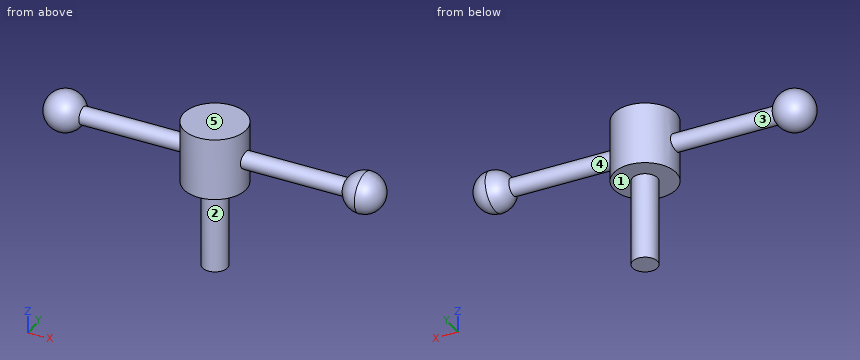
from build123d import *

# Parameters (mm, degrees)
F0_R     = 15.875
F1_DEPTH = 31.75
F2_R     = 6.35
F3_DEPTH = 44.45
F4_R     = 4.445
F5_DEPTH = 76.2


with BuildPart() as f1:
    # F0 (on Top) → F1 (new body)
    with BuildSketch(Plane.XY):
        Circle(F0_R)
    extrude(amount=F1_DEPTH)

    # F2 (on face) → F3 (join)
    with BuildSketch(Plane(origin=(0, 0, 0), x_dir=(1, 0, 0), z_dir=(0, 0, -1))):
        Circle(F2_R)
    extrude(amount=F3_DEPTH)

    # F4 (on Right) → F5 (join, symmetric)
    with BuildSketch(Plane.YZ):
        with Locations((0, 15.875)):
            Circle(F4_R)
    extrude(amount=F5_DEPTH, both=True)

    # F6 (on Front) → F7 (revolve)
    with BuildSketch(Plane.XZ):
        with BuildLine():
            Line((-76.2, 15.875), (-76.2, 20.32))
            Line((-76.2, 20.32), (-67.063941, 20.32))
            ThreePointArc((-67.063941, 20.32), (-78.480706, 25.775706), (-86.36, 15.875))
            Line((-86.36, 15.875), (-76.2, 15.875))
        make_face()
        with BuildLine():
            Line((76.2, 26.035), (76.2, 20.32))
            Line((76.2, 20.32), (76.2, 15.875))
            Line((76.2, 15.875), (86.36, 15.875))
            ThreePointArc((86.36, 15.875), (83.384205, 23.059205), (76.2, 26.035))
        make_face()
        with BuildLine():
            ThreePointArc((76.2, 26.035), (70.811846, 24.488559), (67.063941, 20.32))
            Line((67.063941, 20.32), (76.2, 20.32))
            Line((76.2, 20.32), (76.2, 26.035))
        make_face()
    revolve(axis=Axis((-81.28, 0, 15.875), (1, 0, 0)))


solid = f1.part
For this review, take the finished solid that the model builds, in its own axes (mm). Face numbers are marked on the shaded views. A direction names the side the tool comes from. Round coordinates to 2 decimals unless told otherwise and drop trailing zeros. Write each loop counter-clockwise with the first axis right and the second up, starting at its lowest first coordinate (ties: lowest second). Pieces come first, ordered by that corner, then holes. Notation, with made-up numbers: (10.25, -25) -> (32.25, -25) arc R37 cw to (32.25, 11) -> close; hole circle Ø3 at (-31.5, 38.25). An arc over 180 degrees is marked (long way). Put each result on its own line as item: value.
Q1. Consider section B-B on z = 3. State the section outline as (x, y) points (3 decimals), and give its area (3 significant figures).
Determined:
outline: circle Ø31.75 at (0, 0)
area: 792 mm^2
Q2. Consider section D-D on x = -39.5. State the section outline as (y, z) points (3 decimals).
Determined:
outline: circle Ø8.89 at (0, 15.875)
Q3. Clearance check with flat-ended pins moving along their axes: pin 1 Ø10 at (x, y) = (63.5, -3.5) entering from +Z; pin 2 Ø10 at (x, y) = (-54, 9) entering from -Z; pin 3 Ø2 at (y, z) = (2, 3) entering from -X. State where each tip first meets the part, or that it passes through.
Determined:
pin 1: stops at z = 21.91
pin 2: stops at z = 13.94
pin 3: stops at x = -15.84
Q4. Consider section C-C on y = 8.5. Give the number of separate pieces and of enclosed holes in the cut face, and give its area (3 significant figures).
Determined:
separate pieces: 3
enclosed holes: 0
area: 1,050 mm^2
Q5. The part is to be moulded in two halves that separate along X. For the marked faces 1, 2 and 3, say which applies: released by +X, released by -X, zero draft, split by the parting line, or undercut.
Determined:
face 1: zero draft
face 2: split by the parting line
face 3: undercut
Q6. Consider section A-A on x = 0. State the section outline as (y, z) points (3 decimals), and give its area (3 significant figures).
Determined:
outline: (-15.875, 0) -> (-6.35, 0) -> (-6.35, -44.45) -> (6.35, -44.45) -> (6.35, 0) -> (15.875, 0) -> (15.875, 31.75) -> (-15.875, 31.75) -> close
area: 1,570 mm^2
Q7. To check wall thickness, follow L1, parallel to X at y = 8, z = 15.5; L2, parallel to Z at x = 10, y = -3.5; L3, parallel to X at y = -0.5, z = 9. State the ranges of each line that lie inside material, in increasing order. Write a range as [from, to].
Determined:
L1: x = [-82.45, -69.95], [-13.71, 13.71], [69.95, 82.45]
L2: z = [0, 31.75]
L3: x = [-83.66, -68.74], [-15.87, 15.87], [68.74, 83.66]
Q8. Machinability: for the marked faces 4 and 5, which of the approach directions +Z, -Z, +X, -X, +Y, -Y give a long, thin tool a straight path to every point of the face, cutting with its end or side? Answer none if there is none.
Determined:
face 4: none
face 5: +Z, +X, -X, +Y, -Y
